Can you work these out from the model? Positions are in its coordinate system, mm. Face numbers are marked on the shaded views. A direction names the side the tool comes from. Round coordinates to 2 decimals unless told otherwise and drop trailing zeros. Order: outer loops, then holes, each group sorted by start corner. A loop starts at its lowest first (then second) coordinate and runs counter-clockwise, first axis right, second up. Notation, with made-up numbers: (74, -17.75) -> (80, -17.75) arc R22 cw to (80, 4.25) -> close; hole circle Ø4 at (-2.75, -3). An arc over 180 degrees is marked (long way). One line per item, written item: value.
```python
from build123d import *

# Parameters (mm, degrees)
SKETCH_1_W      = 8.6
SKETCH_1_H      = 4.5
EXTRUDE_1_DEPTH = 4.7
SKETCH_2_W      = 2
SKETCH_2_H      = 2
EXTRUDE_2_DEPTH = 3
SKETCH_4_W      = 0.4
SKETCH_4_H      = 1.2
EXTRUDE_3_DEPTH = 3.1
SKETCH_5_W      = 0.5
SKETCH_5_H      = 0.3
EXTRUDE_4_DEPTH = 3.1


with BuildPart() as part:
    # 草图1 → 凸台-拉伸1 (new body)
    with BuildSketch(Plane(origin=(0, 0, 0), x_dir=(1, 0, 0), z_dir=(0, 1, 0))):
        with Locations((4.3, 2.25)):
            Rectangle(SKETCH_1_W, SKETCH_1_H)
    extrude(amount=EXTRUDE_1_DEPTH)

    # 草图2 → 凸台-拉伸2 (add)
    with BuildSketch(Plane.XY):
        with Locations((3.3, 2.7)):
            Rectangle(SKETCH_2_W, SKETCH_2_H)
    extrude(amount=EXTRUDE_2_DEPTH)

    # 草图4 → 凸台-拉伸3 (add)
    with BuildSketch(Plane.XZ):
        with Locations((0.2, -2.25)):
            Rectangle(SKETCH_4_W, SKETCH_4_H)
        with Locations((8.4, -2.25)):
            Rectangle(SKETCH_4_W, SKETCH_4_H)
    extrude(amount=EXTRUDE_3_DEPTH)

    # 草图5 → 凸台-拉伸4 (add)
    with BuildSketch(Plane.XZ):
        with Locations((4.3, -2.25)):
            Rectangle(SKETCH_5_W, SKETCH_5_H)
        with Locations((6.3, -2.25)):
            Rectangle(SKETCH_5_W, SKETCH_5_H)
        with Locations((2.3, -2.25)):
            Rectangle(SKETCH_5_W, SKETCH_5_H)
    extrude(amount=EXTRUDE_4_DEPTH)


solid = part.part
```
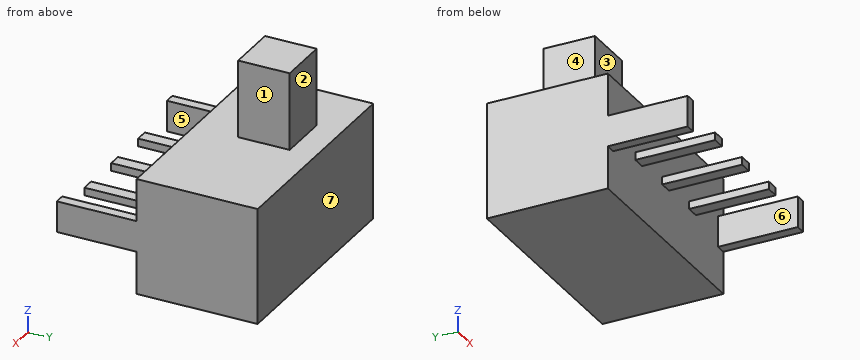
Q1. I want a section at A-A on y = -0.5. List the corners of the cut face in (x, z) for me.
Answers below:
outline: (0, -2.85) -> (0.4, -2.85) -> (0.4, -1.65) -> (0, -1.65) -> close; (2.05, -2.4) -> (2.55, -2.4) -> (2.55, -2.1) -> (2.05, -2.1) -> close; (4.05, -2.4) -> (4.55, -2.4) -> (4.55, -2.1) -> (4.05, -2.1) -> close; (6.05, -2.4) -> (6.55, -2.4) -> (6.55, -2.1) -> (6.05, -2.1) -> close; (8.2, -2.85) -> (8.6, -2.85) -> (8.6, -1.65) -> (8.2, -1.65) -> close
Q2. On a 3-axis mill with a long thin cutter (end or side, diameter ignored), from which of +Z, -Z, +X, -X, +Y, -Y can I reach the whole of each face in a straight line? I mean the marked faces 1, 2 and 3. Say none if no direction works.
Answers below:
face 1: +Z, +X, +Y, -Y
face 2: +Z, +X, -X, +Y
face 3: +Z, +X, -X, -Y
Q3. Will these pins go through, and if not, where does the flat tip stop? pin 1 Ø0.6 at (x, z) = (3, 1.5) entering from -Y; pin 2 Ø1.6 at (y, z) = (2.5, 1) entering from +X; pin 3 Ø0.6 at (x, y) = (4.5, -1) entering from +Z.
Answers below:
pin 1: y = 1.7
pin 2: x = 4.3
pin 3: z = -2.1
Q4. I want a section at B-B on y = 3.5. List the corners of the cut face in (x, z) for me.
Answers below:
outline: (0, -4.5) -> (8.6, -4.5) -> (8.6, 0) -> (4.3, 0) -> (4.3, 3) -> (2.3, 3) -> (2.3, 0) -> (0, 0) -> close
Q5. Please list where these lines run through material, in increasing order: line 1 along Y through (x, z) = (6.5, -2.5); line 2 along Z through (x, y) = (1.25, 2).
Answers below:
line 1: 0 to 4.7
line 2: -4.5 to 0
Q6. We'd pull the mould along X, two halves only. Please class the marked faces 4, 5, 6 and 7: released by +X, released by -X, zero draft, split by the parting line, or undercut.
Answers below:
face 4: released by -X
face 5: undercut
face 6: undercut
face 7: zero draft
Q7. I want a section at C-C on x = 6.25. List the corners of the cut face in (y, z) for me.
Answers below:
outline: (-3.1, -2.4) -> (0, -2.4) -> (0, -4.5) -> (4.7, -4.5) -> (4.7, 0) -> (0, 0) -> (0, -2.1) -> (-3.1, -2.1) -> close
Q8. I want a section at D-D on z = 2.75. List the corners of the cut face in (x, y) for me, plus the area to 3 significant figures.
Answers below:
outline: (2.3, 1.7) -> (4.3, 1.7) -> (4.3, 3.7) -> (2.3, 3.7) -> close
area: 4.00 mm^2
